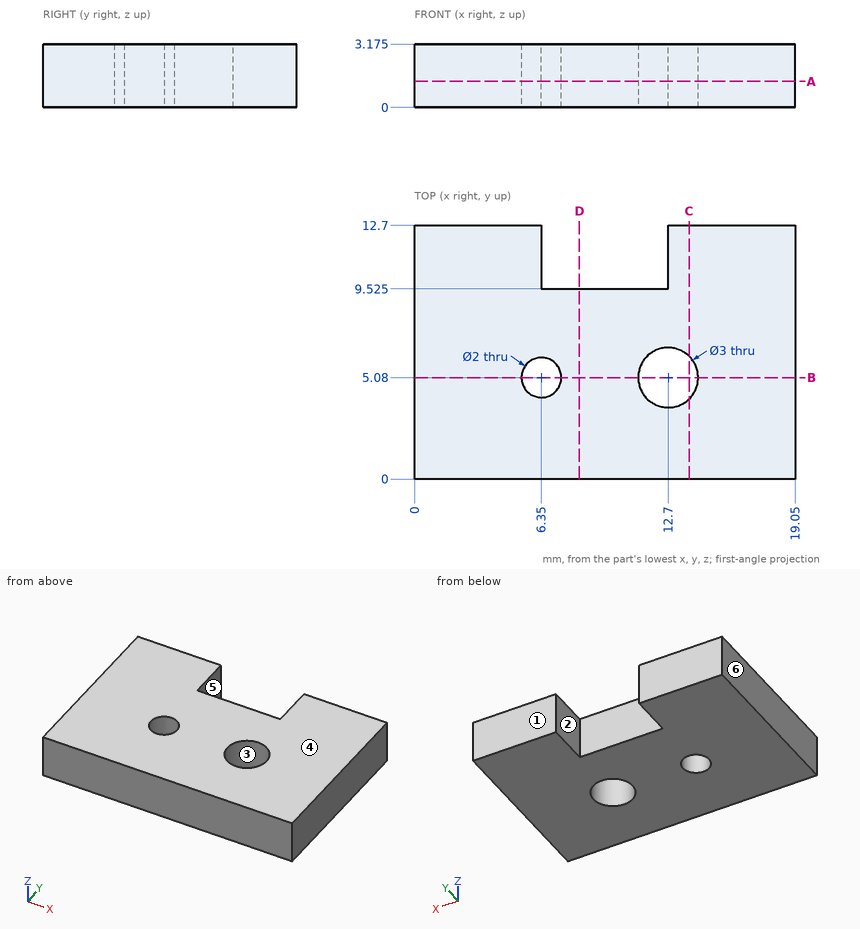
Here's the drawing with two shaded views (mm, measured from the low corner). I have some questions. A direction names the side the tool comes from. Coordinates: 2 decimals unless noted, no trailing zeros. Loops run counter-clockwise (first coordinate to the right, second up) from the corner with the lowest first, then second, coordinate; pieces in that order, holes last. Notation, with made-up numbers: (35, 25) -> (88, 25) arc R13 ccw to (88, 30) -> close; hole circle Ø3 at (-6.5, 70.5). An arc over 180 degrees is marked (long way). Use one line per item in the form item = value. Start each with the question number.
(1) If we section it at B-B (y = 5.08): Please give me the cut outline in (x, z) (3 decimals), then the cut area to 3 significant figures.
(2) If we section it at C-C (x = 13.75): Please give me the cut outline in (y, z) (3 decimals).
(3) On a 3-axis mill with a long thin cutter (end or side, diameter ignored), from which of +Z, -Z, +X, -X, +Y, -Y can I reach the whole of each face in a straight line? I mean the marked faces 1 and 2. Say none if no direction works.
(4) If we section it at A-A (z = 1.3): Please give me the cut outline in (x, y) (3 decimals).
(5) Please list where these lines run through material, in increasing order: line 1 along X through (y, z) = (5.75, 2.3); line 2 along X through (y, z) = (10.5, 1.05); line 3 along Y through (x, z) = (8.75, 0.35) (3 decimals).
(6) We'd pull the mould along X, two halves only. Please class the marked faces 3, 4, 5 and 6: pulls with the +X half, pulls with the -X half, needs draft (parallel to the pull), parting line crosses it, or undercut.
(7) If we section it at D-D (x = 8.25): Please give me the cut outline in (y, z) (3 decimals), then the cut area to 3 significant figures.
(8) Will these pins go through, and if not, where does the flat tip stop? pin 1 (3 mm diameter, centred on x = 16, y = 6.5, fed in from -Z); pin 2 (1.6 mm diameter, centred on x = 6.35, y = 5.08, fed in from +Z).
Verdict:
q1.outline = (0, 0) -> (5.35, 0) -> (5.35, 3.175) -> (0, 3.175) -> close; (7.35, 0) -> (11.2, 0) -> (11.2, 3.175) -> (7.35, 3.175) -> close; (14.2, 0) -> (19.05, 0) -> (19.05, 3.175) -> (14.2, 3.175) -> close
q1.area = 44.6 mm²
q2.outline = (0, 0) -> (4.009, 0) -> (4.009, 3.175) -> (0, 3.175) -> close; (6.151, 0) -> (12.7, 0) -> (12.7, 3.175) -> (6.151, 3.175) -> close
q3.face_1 = +Z, -Z, +X, -X, +Y
q3.face_2 = +Z, -Z, +Y
q4.outline = (0, 0) -> (19.05, 0) -> (19.05, 12.7) -> (12.7, 12.7) -> (12.7, 9.525) -> (6.35, 9.525) -> (6.35, 12.7) -> (0, 12.7) -> close; hole circle Ø2 at (6.35, 5.08); hole circle Ø3 at (12.7, 5.08)
q5.line_1 = 0 to 5.61, 7.09 to 11.36, 14.04 to 19.05
q5.line_2 = 0 to 6.35, 12.7 to 19.05
q5.line_3 = 0 to 9.525
q6.face_3 = undercut
q6.face_4 = needs draft
q6.face_5 = undercut
q6.face_6 = pulls with the -X half
q7.outline = (0, 0) -> (9.525, 0) -> (9.525, 3.175) -> (0, 3.175) -> close
q7.area = 30.2 mm²
q8.pin_1 = 0
q8.pin_2 = through
